Input: part model. Units: mm. Frame: model coordinates. A direction names the side the tool comes from. Give positions to 0.01 mm unless a question says otherwise; leave off trailing zeros. Loops run counter-clockwise (first coordinate to the right, second up) from the corner with the lowest first, then second, coordinate; pieces in that order, holes last. Notation, with made-up numbers: (3, 18) -> (20, 18) arc R28 cw to (20, 39) -> close; hole circle Ø2 at (74.25, 55.5). An arc over 180 degrees is marked (long way). One line per question, with ' | ' between items.
Autodesk Fusion 360 part; units mm, degrees
sketch "Sketch1" plane through (0, 0, 0) normal (0, 0, 1) x (1, 0, 0)
  line L0 (13.85, 9) -> (-13.85, 9) construction
  line L1 (-13.85, 9) -> (-13.85, -9) construction
  line L2 (-13.85, -9) -> (13.85, -9) construction
  line L3 (13.85, -9) -> (13.85, 9) construction
  line L4 (13.85, 9) -> (-13.85, -9) construction
  line L5 (-13.85, 9) -> (13.85, -9) construction
  line L6 (-11.25, 8) -> (11.25, 8)
  line L7 (11.25, 8) -> (11.25, -5.4)
  line L8 (11.25, -5.4) -> (-11.25, -5.4)
  line L9 (-11.25, -5.4) -> (-11.25, 8)
  circle A0 centre (0, 0) radius 3.5
  line L10 (2.4, -0.6) -> (-2.4, -0.6)
  line L11 (-2.4, -0.6) -> (-2.4, 0.6)
  line L12 (-2.4, 0.6) -> (2.4, 0.6)
  line L13 (2.4, 0.6) -> (2.4, -0.6)
  line L14 (2.4, -0.6) -> (-2.4, 0.6) construction
  line L15 (-2.4, -0.6) -> (2.4, 0.6) construction
  line L16 (0.6, -2.4) -> (-0.6, -2.4)
  line L17 (-0.6, -2.4) -> (-0.6, 2.4)
  line L18 (-0.6, 2.4) -> (0.6, 2.4)
  line L19 (0.6, 2.4) -> (0.6, -2.4)
  line L20 (0.6, -2.4) -> (-0.6, 2.4) construction
  line L21 (-0.6, -2.4) -> (0.6, 2.4) construction
  line L22 (-0.6, 2.4) -> (-2.5475, 2.4)
  line L23 (0.6, 2.4) -> (2.5475, 2.4)
  line L24 (-0.6, -2.4) -> (-2.5475, -2.4)
  line L25 (0.6, -2.4) -> (2.5475, -2.4)
  dimension "d1" = 27.7
  dimension "d2" = 18
  dimension "d3" = 3.6
  dimension "d4" = 1
  dimension "d5" = 2.6
  dimension "d6" = 2.6
  dimension "d7" = 7
  dimension "d8" = 4.8
  dimension "d9" = 1.2
  dimension "d10" = 1.2
  dimension "d11" = 4.8
extrude "Extrude1" add sketch "Sketch1" along normal blind 0.6 contours L6 L7 L8 L9 | A0 L10 L12 L13 L19 L23 L25 | A0 L18 L22 L23 | A0 L16 L24 L25 | A0 L10 L11 L12 L17 L22 L24 | L12 L17 L18 L19 | L10 L16 L17 L19 | L10 L12 L17 L19 | L10 L12 L13 L19 | L10 L11 L12 L17
extrude "Extrude2" add sketch "Sketch1" along normal blind 4 contours A0 L10 L12 L13 L19 L23 L25 | A0 L10 L11 L12 L17 L22 L24
fillet "Fillet1" radius 1 6 edges at (-1.5738, -2.4, 0.6) (-3.5, 0, 0.6) (1.5738, -2.4, 0.6) (3.5, 0, 0.6) (1.5738, 2.4, 0.6) (-1.5738, 2.4, 0.6)
fillet "Fillet1" radius 0.5 4 edges at (11.25, 8, 0.3) (-11.25, 8, 0.3) (11.25, -5.4, 0.3) (-11.25, -5.4, 0.3)
chamfer "Chamfer1" distance 0.4 angle 45 20 edges at (-11.1036, 7.8536, 0) (0, 8, 0) (11.1036, 7.8536, 0) (11.25, 1.3, 0) (11.1036, -5.2536, 0) (0, -5.4, 0) (-11.1036, -5.2536, 0) (-11.25, 1.3, 0) (-0.6, 1.5, 4) (-1.5, 0.6, 4) (-2.4, 0, 4) (-1.5, -0.6, 4) (-0.6, -1.5, 4) (0.6, -1.5, 4) (1.5, -0.6, 4) (2.4, 0, 4) (1.5, 0.6, 4) (0.6, 1.5, 4) (3.5, 0, 4) (-3.5, 0, 4)
1. Section query B-B (x = 5.5). Output: boundary loops of the cut face in (y, z).
Determined:
outline: (-5.4, 0.4) -> (-5, 0) -> (7.6, 0) -> (8, 0.4) -> (8, 0.6) -> (-5.4, 0.6) -> close
2. Section query C-C (y = 4). Output: boundary loops of the cut face in (x, z).
Determined:
outline: (-11.25, 0.4) -> (-10.85, 0) -> (10.85, 0) -> (11.25, 0.4) -> (11.25, 0.6) -> (-11.25, 0.6) -> close
3. Ray query, line 1 along Z through (x, y) = (-5, -2); line 2 along X through (y, z) = (0.75, 2.7); line 3 along X through (y, z) = (-0.75, 0.9). Return the intervals inside material, ascending. Write a range as from..to.
Determined:
line 1: z = 0..0.6 | line 2: x = -3.42..-0.6, 0.6..3.42 | line 3: x = -3.71..-0.6, 0.6..3.71
4. Pull-direction query (Y, two-part tool) for faces 1 (the conical face through (-3.21, -0.04, 3.89)), 2 (the flat face through (-0.6, 2, 2)), 3 (the flat face through (-1, -0.6, 2)); classes: pulls with the +Y half, pulls with the -Y half, needs draft (parallel to the pull), parting line crosses it, or undercut.
Determined:
face 1: parting line crosses it | face 2: needs draft | face 3: undercut
5. Section query A-A (z = 2). Output: boundary loops of the cut face in (x, y).
Determined:
outline: (-2.55, -2.4) -> (-0.6, -2.4) -> (-0.6, -0.6) -> (-2.4, -0.6) -> (-2.4, 0.6) -> (-0.6, 0.6) -> (-0.6, 2.4) -> (-2.55, 2.4) arc R3.5 ccw to start; (0.6, -2.4) -> (2.55, -2.4) arc R3.5 ccw to (2.55, 2.4) -> (0.6, 2.4) -> (0.6, 0.6) -> (2.4, 0.6) -> (2.4, -0.6) -> (0.6, -0.6) -> close
6. Section query D-D (z = 0.9). Output: boundary loops of the cut face in (x, y), then the cut area to 3 significant figures.
Determined:
outline: (-2.67, -2.69) -> (-0.6, -2.69) -> (-0.6, -0.6) -> (-2.4, -0.6) -> (-2.4, 0.6) -> (-0.6, 0.6) -> (-0.6, 2.69) -> (-2.67, 2.69) arc R3.79 ccw to start; (0.6, -2.69) -> (2.67, -2.69) arc R3.79 ccw to (2.67, 2.69) -> (0.6, 2.69) -> (0.6, 0.6) -> (2.4, 0.6) -> (2.4, -0.6) -> (0.6, -0.6) -> close | area: 26.2 mm2
7. Reachability of faces 4 (the cylindrical face through (-3.5, 0, 2.6)), 5 (the flat face through (2, -2.4, 3)), 6 (the flat face through (-2.4, 0, 2)) from +Z, -Z, +X, -X, +Y, -Y: full face, straight path, thin tool, end or side. Return the list, or none.
Determined:
face 4: +Z, -X | face 5: +Z, +X, -X, -Y | face 6: +Z
8. Pin query (flat end, axial travel): P1, Ø0.6, axis at x = 2, z = 3.5, coming from the +Y side; P2, Ø0.6, axis at y = 0.5, z = 2.5, coming from the -X side; P3, Ø1.5, axis at y = -3, z = 2.5, coming from the +X side. Return the tip coordinate at first contact, or that it passes through.
Determined:
P1: stops at y = 2.4 | P2: stops at x = -3.49 | P3: stops at x = 2.68
